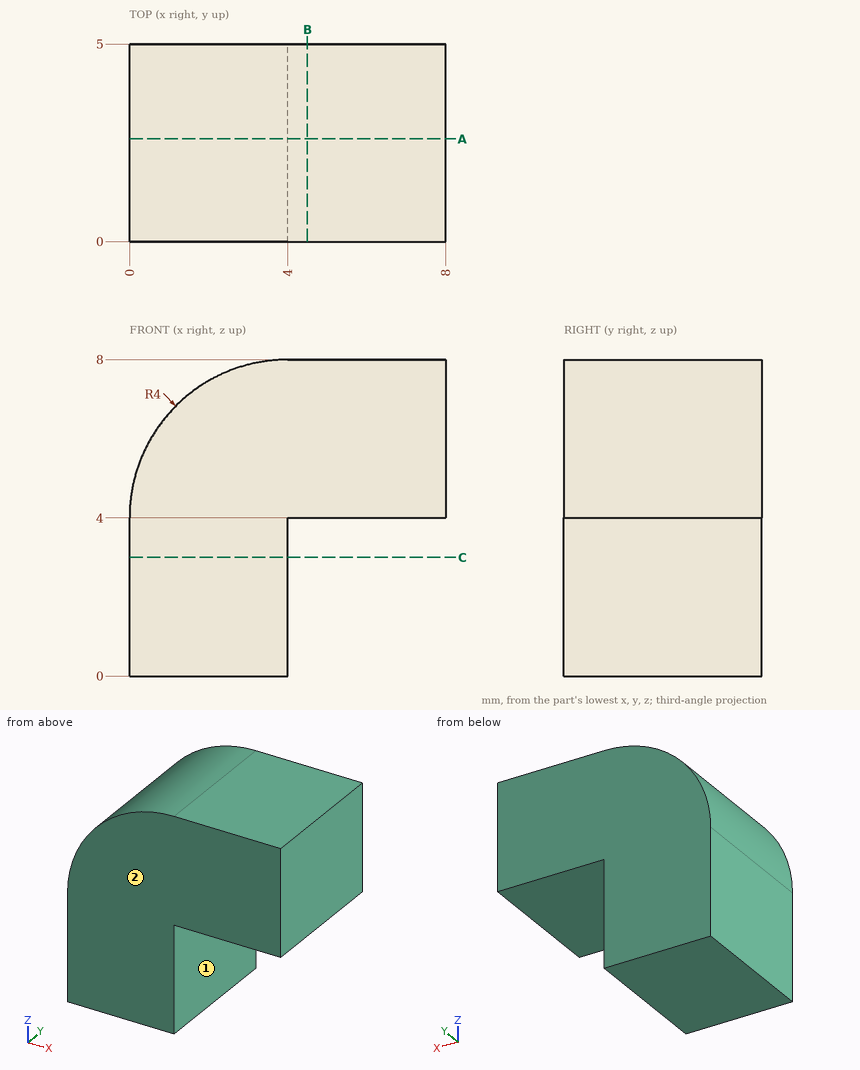
Design review of the part shown in the three views and the two pictorial views. Dimensions are in mm from the part's minimum x, y and z. A direction names the side the tool comes from. Give positions to 0.01 mm unless a question says otherwise; leave off trailing zeros. Write each loop counter-clockwise with the first axis right and the second up, starting at its lowest first coordinate (ties: lowest second). Pieces come first, ordered by that corner, then holes. Notation, with made-up numbers: M -0.5,6.25 L 28.5,6.25 A25 cw 28.5,45.25 Z; hole C -5,60 d6. An arc over 180 degrees is marked long. Return JSON: item names as keys, results as strings. Group by question number.
Item 1: Wall thickness on line 1 along X through (y, z) = (3.45, 2.5); line 2 along Z through (x, y) = (6.25, 3.45); line 3 along Z through (x, y) = (0.5, 2.15): over which ranges is each line inside the solid? List them lowest first.
Item 2: Clearance check with a flat-ended pin moving along its axis: pin 1 Ø3 at (y, z) = (2.5, 2) entering from +X. State where the tip first meets the part, or that it passes through.
Item 3: Tool access review of the marked faces 1 and 2: name each direction out of +Z, -Z, +X, -X, +Y, -Y from which nothing blocks a thin tool from reaching the whole face with its end or side.
Item 4: Take a section at A-A (y = 2.6). Give the boundary of the cut face in (x, z), plus the area to 3 significant figures.
Item 5: Take a section at B-B (x = 4.5). Give the boundary of the cut face in (y, z), plus the area to 3 significant figures.
Item 6: Take a section at C-C (z = 3). Give the boundary of the cut face in (x, y), plus the area to 3 significant figures.
Return value:
{
 "1": {"line 1": "x = 0 to 4", "line 2": "z = 4 to 8", "line 3": "z = 0 to 5.94"},
 "2": {"pin 1": "stops at x = 4"},
 "3": {"face 1": "-Z, +X, +Y, -Y", "face 2": "+Z, -Z, +X, -X, -Y"},
 "4": {"outline": "M 0,0 L 4,0 L 4,4 L 8,4 L 8,8 L 4,8 A4 ccw 0,4 Z", "area": "44.6 mm2"},
 "5": {"outline": "M 0,4 L 5,4 L 5,8 L 0,8 Z", "area": "20.0 mm2"},
 "6": {"outline": "M 0,0 L 4,0 L 4,5 L 0,5 Z", "area": "20.0 mm2"}
}
